Geometry: final body of the model. Coordinates: model frame, mm. Face numbers are marked on the shaded views. A direction names the side the tool comes from. Give positions to 0.01 mm unless a question says otherwise; leave off trailing zeros. Order: outer loops, then holes, each group sorted by start corner. A loop starts at its lowest first (then second) coordinate and runs counter-clockwise, first axis right, second up. Notation, with made-up numbers: (-1, 19.5) - (17, 19.5) arc R19 ccw to (17, 49.5) - close; hole circle Ø5 at (84.5, 16). An arc over 180 degrees is marked (long way). One line per item, written item: value.
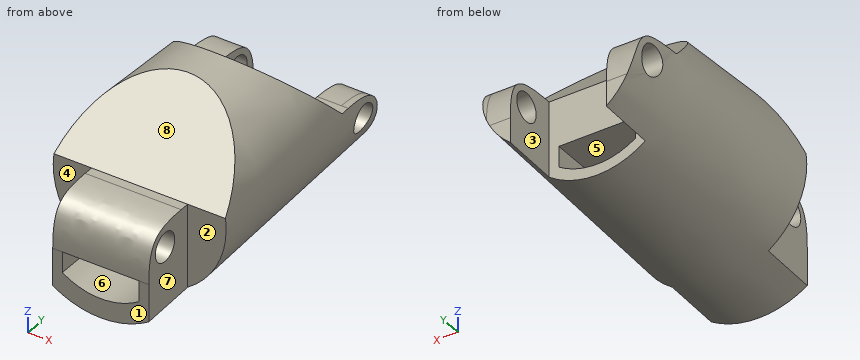
```python
from build123d import *

# Parameters (mm, degrees)
SKETCH1_R                     = 9
BOSS_EXTRUDE1_DEPTH           = 25
BOSS_EXTRUDE1_TAPER           = 2
BOSS_EXTRUDE1_OTHER_WAY_DEPTH = 6
BOSS_EXTRUDE1_OTHER_WAY_TAPER = -2
CUT_EXTRUDE1_DEPTH            = 29.189194514
CUT_EXTRUDE1_DEPTH_BACK       = 29.189194514
CUT_EXTRUDE2_START            = -10.365035118
CUT_EXTRUDE2_OUTLINE_W        = 9.770566763
CUT_EXTRUDE2_OUTLINE_H        = 6
CUT_EXTRUDE2_DEPTH            = 10.365035118
CUT_EXTRUDE3_DEPTH            = 31.096766332
CUT_EXTRUDE3_DEPTH_BACK       = 31.096766332
SKETCH5_R                     = 1.5
FILLET1_SIZE                  = 5
CUT_EXTRUDE4_DEPTH            = 29.121439218
CUT_EXTRUDE4_DEPTH_BACK       = 29.121439218
SKETCH8_W                     = 10
SKETCH8_H                     = 6
CUT_EXTRUDE5_DEPTH            = 29.520763505
CUT_EXTRUDE6_DEPTH            = 31.096766332
CUT_EXTRUDE6_DEPTH_BACK       = 31.096766332
SKETCH9_R                     = 1.5
FILLET2_SIZE                  = 5
CUT_EXTRUDE7_DEPTH            = 34.568070447


with BuildPart() as part:
    # Sketch1 → Boss-Extrude1 (new body)
    with BuildSketch(Plane(origin=(0, 0, 0), x_dir=(1, 0, 0), z_dir=(0, 1, 0))):
        Circle(SKETCH1_R)
    extrude(amount=BOSS_EXTRUDE1_DEPTH, taper=BOSS_EXTRUDE1_TAPER)

    # Sketch1 → Boss-Extrude1 other way (add)
    with BuildSketch(Plane(origin=(0, 0, 0), x_dir=(1, 0, 0), z_dir=(0, 1, 0))):
        Circle(SKETCH1_R)
    extrude(amount=-BOSS_EXTRUDE1_OTHER_WAY_DEPTH, taper=BOSS_EXTRUDE1_OTHER_WAY_TAPER)

    # Sketch3 → Cut-Extrude1 (cut, two sides: drawn at the far end of the back side and taken through both)
    with BuildSketch(Plane(origin=(0, 0, 0), x_dir=(0, 0, -1), z_dir=(1, 0, 0)).offset(-CUT_EXTRUDE1_DEPTH_BACK)):
        Polygon((-1.155510401, -6), (-1.155510401, 0), (-11.155510401, 10), (-11.155510401, -6), align=None)
    extrude(amount=CUT_EXTRUDE1_DEPTH + CUT_EXTRUDE1_DEPTH_BACK, mode=Mode.SUBTRACT)

    # Cut-Extrude2: read off the stored shape, not the designer's step
    # Cut-Extrude2 outline → Cut-Extrude2 (cut)
    with BuildSketch(Plane.XY.offset(1.155510401).offset(CUT_EXTRUDE2_START)):
        with Locations((-9.885283382, -3)):
            Rectangle(CUT_EXTRUDE2_OUTLINE_W, CUT_EXTRUDE2_OUTLINE_H)
        with Locations((9.885283382, -3)):
            Rectangle(CUT_EXTRUDE2_OUTLINE_W, CUT_EXTRUDE2_OUTLINE_H)
    extrude(amount=CUT_EXTRUDE2_DEPTH, mode=Mode.SUBTRACT)

    # Sketch5 → Cut-Extrude3 (cut, two sides: drawn at the far end of the back side and taken through both)
    with BuildSketch(Plane.ZY.offset(5).offset(-CUT_EXTRUDE3_DEPTH_BACK)):
        with Locations(Location((-1.344489599, -3.5, 0), (0, 0, 270))):
            Circle(SKETCH5_R)
    extrude(amount=CUT_EXTRUDE3_DEPTH + CUT_EXTRUDE3_DEPTH_BACK, mode=Mode.SUBTRACT)

    # Fillet1
    # a fillet whose section is not a circle: 5 mm, written as the material it takes off along each edge
    with BuildSketch(Plane(origin=(17.5, -6, 1.155510401), x_dir=(0, 0, -1), z_dir=(-1, 0, 0))) as fillet1_piece_1:
        with BuildLine():
            Bezier((FILLET1_SIZE, 0), (0, 0), (0, -FILLET1_SIZE), weights=[1, 1.5, 1])
            Line((0, -FILLET1_SIZE), (0, 0))
            Line((0, 0), (FILLET1_SIZE, 0))
        make_face()
    extrude(amount=35, mode=Mode.SUBTRACT)

    # Sketch7 → Cut-Extrude4 (cut, two sides: drawn at the far end of the back side and taken through both)
    with BuildSketch(Plane(origin=(0, 0, 0), x_dir=(0, 0, -1), z_dir=(1, 0, 0)).offset(-CUT_EXTRUDE4_DEPTH_BACK)):
        Polygon((-1.155510401, 25), (-1.155510401, 19), (-12.24506556, 7.91044484), (-12.24506556, 25), align=None)
    extrude(amount=CUT_EXTRUDE4_DEPTH + CUT_EXTRUDE4_DEPTH_BACK, mode=Mode.SUBTRACT)

    # Sketch8 → Cut-Extrude5 (cut, through all)
    with BuildSketch(Plane.XY.offset(1.155510401)):
        with Locations((0, 22)):
            Rectangle(SKETCH8_W, SKETCH8_H)
    extrude(amount=-CUT_EXTRUDE5_DEPTH, mode=Mode.SUBTRACT)

    # Sketch9 → Cut-Extrude6 (cut, two sides: drawn at the far end of the back side and taken through both)
    with BuildSketch(Plane(origin=(-5, 0, 0), x_dir=(0, 0, -1), z_dir=(1, 0, 0)).offset(-CUT_EXTRUDE6_DEPTH_BACK)):
        with Locations(Location((1.344489599, 22.5, 0), (0, 0, 311.001081294))):
            Circle(SKETCH9_R)
    extrude(amount=CUT_EXTRUDE6_DEPTH + CUT_EXTRUDE6_DEPTH_BACK, mode=Mode.SUBTRACT)

    # Fillet2
    # a fillet whose section is not a circle: 5 mm, written as the material it takes off along each edge
    with BuildSketch(Plane(origin=(-20.544414959, 25, 1.155510401), x_dir=(0, 0, -1), z_dir=(1, 0, 0))) as fillet2_piece_1:
        with BuildLine():
            Bezier((FILLET2_SIZE, 0), (0, 0), (0, -FILLET2_SIZE), weights=[1, 1.5, 1])
            Line((0, -FILLET2_SIZE), (0, 0))
            Line((0, 0), (FILLET2_SIZE, 0))
        make_face()
    extrude(amount=28.044414959, mode=Mode.SUBTRACT)
    with BuildSketch(Plane(origin=(-7.5, 25, 1.155510401), x_dir=(0, -1, 0), z_dir=(1, 0, 0))) as fillet2_piece_2:
        with BuildLine():
            Bezier((FILLET2_SIZE, 0), (0, 0), (0, FILLET2_SIZE), weights=[1, 1.5, 1])
            Line((0, FILLET2_SIZE), (0, 0))
            Line((0, 0), (FILLET2_SIZE, 0))
        make_face()
    extrude(amount=28.044414959, mode=Mode.SUBTRACT)

    # Sketch10 → Cut-Extrude7 (cut, through all)
    with BuildSketch(Plane.XZ.offset(6)):
        with BuildLine():
            Line((-4, -3.844489599), (-4, -5.998103467))
            ThreePointArc((-4, -5.998103467), (0, -7.209524617), (4, -5.998103467))
            Line((4, -5.998103467), (4, -3.844489599))
            Line((4, -3.844489599), (-4, -3.844489599))
        make_face()
    extrude(amount=-CUT_EXTRUDE7_DEPTH, mode=Mode.SUBTRACT)


solid = part.part
```
1) Mould query, pull axis X, two halves, no side actions, for the marked faces 6, 7 and 8. Classes: released by +X, released by -X, zero draft, split by the parting line, or undercut.
Answers below:
face 6: undercut
face 7: released by +X
face 8: zero draft
2) Set-up query: the marked faces 1, 2, 3, 4 and 5. Return all of +Z, -Z, +X, -X, +Y, -Y with unobstructed straight access to the full face (end or side cutting, diameter ignored); none if empty.
Answers below:
face 1: +Z, -Z, +X, -X, -Y
face 2: +Z, -Z, +X, -Y
face 3: +Z, -Z, +Y
face 4: +Z, -Z, -X, -Y
face 5: +Y, -Y
3) First-contact query: pin 1 (1 mm diameter, centred on x = -7, y = 20.5, fed in from -Z); pin 2 (10 mm diameter, centred on x = 7, y = -2, fed in from -Z); pin 3 (3 mm diameter, centred on x = -7, z = -3, fed in from -Y); pin 4 (10 mm diameter, centred on x = -2, y = 9, fed in from +Z). Flat tips, straight axial feed; report the tip coordinate or a pass-through.
Answers below:
pin 1: z = -5.14
pin 2: z = -8.86
pin 3: y = 0
pin 4: z = 8.74
4) Section A-A, the plane x = -2. Count the separate pieces of the cut face and the enclosed holes in it, then the cut area to 3 significant figures.
Answers below:
separate pieces: 2
enclosed holes: 1
area: 241 mm^2
5) Section C-C, the plane y = 19.5. Return loops of the section in (x, z), then the cut area to 4 significant figures.
Answers below:
outline: (-8.24, 1.16) arc R8.32 ccw to (-5, -6.65) - (-5, 1.16) - close; (5, -6.65) arc R8.32 ccw to (8.24, 1.16) - (5, 1.16) - close
area: 38.45 mm^2
6) Section B-B, the plane y = 4.5. Return loops of the section in (x, z), then the cut area to 3 significant figures.
Answers below:
outline: (-6.8, 5.66) arc R8.84 ccw (long way) to (6.8, 5.66) - close; hole (-4, -6) arc R7.21 ccw to (4, -6) - (4, -3.84) - (-4, -3.84) - close
area: 192 mm^2
7) Material intervals for line 1 along X through (y, z) = (-2, -2); line 2 along Z through (x, y) = (1.75, -3.5); line 3 along Z through (x, y) = (-0.25, -3.5), sorted ascending.
Answers below:
line 1: -5 to 5
line 2: -8.95 to -6.99, -3.84 to -2.84, 0.16 to 0.93
line 3: -9.12 to -7.21, -3.84 to -2.84, 0.16 to 0.93
